from build123d import *

# Parameters (mm, degrees)
BOSS_EXTRUDE1_DEPTH = 10


with BuildPart() as part:
    # Sketch1 → Boss-Extrude1 (new body)
    with BuildSketch(Plane.XY):
        with BuildLine():
            Line((0, 0), (0, 32.5))
            Line((0, 32.5), (3.133753016, 25.7102018))
            Line((3.133753016, 25.7102018), (22.989665666, 38.35981325))
            ThreePointArc((22.989665666, 38.35981325), (36.796576207, 35.298894875), (33.735657833, 21.491984334))
            Line((33.735657833, 21.491984334), (15, 9.556053912))
            ThreePointArc((15, 9.556053912), (13.020876433, 4.778026956), (15, 0))
            Line((15, 0), (0, 0))
        make_face()
    extrude(amount=BOSS_EXTRUDE1_DEPTH)


solid = part.part
Read the model definition and answer for the solid it produces. Units are mm, in the model's axes. A direction names the side the tool comes from. Give positions to 0.01 mm unless a question says otherwise; leave off trailing zeros. Write each loop counter-clockwise with the first axis right and the second up, starting at its lowest first coordinate (ties: lowest second). Pieces come first, ordered by that corner, then holes. Notation, with made-up numbers: M 80,31 L 94,31 A31 cw 94,66 Z; hole C 67.5,-22 d11. An arc over 180 degrees is marked long. One line per item, written item: value. Start each with the question number.
(1) Determine the mould class of faces 1 (the flat face through (0, 16, 5)), 2 (the flat face through (12.923, 31.946, 4.93)), 3 (the flat face through (24.5, 15.61, 4.93)), 4 (the flat face through (8, 0, 5)) for opening direction X: pulls with the +X half, pulls with the -X half, needs draft (parallel to the pull), parting line crosses it, or undercut.
(2) Find section D-D (x = 23.5). Determine the outline of the cut face in (y, z).
(3) Flat-ended cylindrical pins translate along their axes: pin 1 Ø3 at (x, z) = (31, 1.5) entering from +Y; pin 2 Ø1.5 at (y, z) = (32.5, 8) entering from +X. Find the tip coordinate at first contact, or state that the pin passes through.
(4) A tool of negligible diameter and unlimited length cuts with its end or side. For faces 5 (the flat face through (19, 20, 0)), 6 (the flat face through (1.545, 29.153, 4.93)), from which of +Z, -Z, +X, -X, +Y, -Y can it reach the whole face along a straight path? Write none if from no direction.
(5) Find the intervals of material crossed by line 1 (X direction, y = 29, z = 6.25); line 2 (X direction, y = 29.5, z = 4.5); line 3 (Y direction, x = 14, z = 8.5), in increasing order.
(6) Find section C-C (z = 6.5). Determine the outline of the cut face in (x, y), plus the area to 3 significant figures.
(7) Find section B-B (x = 14.5). Determine the outline of the cut face in (y, z).
(8) Find section A-A (y = 29.5). Determine the outline of the cut face in (x, z).
Results below:
1. face 1: pulls with the -X half
1. face 2: undercut
1. face 3: pulls with the +X half
1. face 4: needs draft
2. outline: M 14.97,0 L 38.66,0 L 38.66,10 L 14.97,10 Z
3. pin 1: stops at y = 39.86
3. pin 2: stops at x = 38.19
4. face 5: -Z, +X, -X, +Y, -Y
4. face 6: +Z, -Z, +Y
5. line 1: x = 0 to 1.62, 8.3 to 38.32
5. line 2: x = 0 to 1.38, 9.08 to 38.35
5. line 3: y = 0 to 1.27, 8.28 to 32.63
6. outline: M 0,0 L 15,0 A6.76 cw 15,9.56 L 33.74,21.49 A10 ccw 22.99,38.36 L 3.13,25.71 L 0,32.5 Z
6. area: 902 mm^2
7. outline: M 0,0 L 0.56,0 L 0.56,10 L 0,10 Z; M 9,0 L 32.95,0 L 32.95,10 L 9,10 Z
8. outline: M 0,0 L 1.38,0 L 1.38,10 L 0,10 Z; M 9.08,0 L 38.35,0 L 38.35,10 L 9.08,10 Z
